Build history of the part. All positions in model axes, mm. Round coordinates to 2 decimals unless told otherwise and drop trailing zeros. Write each loop counter-clockwise with the first axis right and the second up, starting at its lowest first coordinate (ties: lowest second). Pieces come first, ordered by that corner, then holes. Notation, with made-up numbers: (57.5, 64) -> (62.5, 64) arc R29 cw to (62.5, 92) -> close; hole circle Ø1 at (-12, -15). An arc over 180 degrees is marked (long way). Answer in a Markdown table with one row per item.
Autodesk Fusion 360 part; units mm, degrees
sketch "8mm circle" plane through (0, 0, 0) normal (0, 0, 1) x (1, 0, 0)
  circle A0 centre (0, 0) radius 4
  dimension "d1" = 8
extrude "Extrude1" add sketch "8mm circle" along normal mid plane 200 makes body 1
copy_body "Body->Comp1" bodies 1 removing the originals makes body 2 in component "8mm shaft"
component "8mm shaft" placed x (1, 0, 0) y (0, 1, 0) z (0, 0, 1) at (0, 0, 0)
Q1. Drop flat-ended pins along their axis: P1, Ø1, axis at x = 2, z = -27, coming from the +Y side; P2, Ø1, axis at y = 1, z = -2, coming from the -X side; P3, Ø1.5, axis at y = -2.5, z = 27, coming from the -X side. Give the stop position or say it passes through.
A:
| item | result |
|---|---|
| P1 | y = 3.71 |
| P2 | x = -3.97 |
| P3 | x = -3.6 |
Q2. Wall check: line 1 (X direction, y = -0.25, z = -31); line 2 (X direction, y = 3, z = -46); line 3 (Y direction, x = 1, z = 39). Give the ranges that are in metal, low to high. Write a range as [from, to].
A:
| item | result |
|---|---|
| line 1 | [-3.99, 3.99] |
| line 2 | [-2.65, 2.65] |
| line 3 | [-3.87, 3.87] |
Q3. Saw through at A-A on z = -37. Write the cut outline in (x, y).
A:
| item | result |
|---|---|
| outline | circle Ø8 at (0, 0) |
Q4. Saw through at B-B on y = -2.5. Write the cut outline in (x, z), plus the area to 3 significant figures.
A:
| item | result |
|---|---|
| outline | (-3.12, -100) -> (3.12, -100) -> (3.12, 100) -> (-3.12, 100) -> close |
| area | 1,250 mm² |
Q5. Saw through at C-C on x = 1.25. Write the cut outline in (y, z).
A:
| item | result |
|---|---|
| outline | (-3.8, -100) -> (3.8, -100) -> (3.8, 100) -> (-3.8, 100) -> close |
